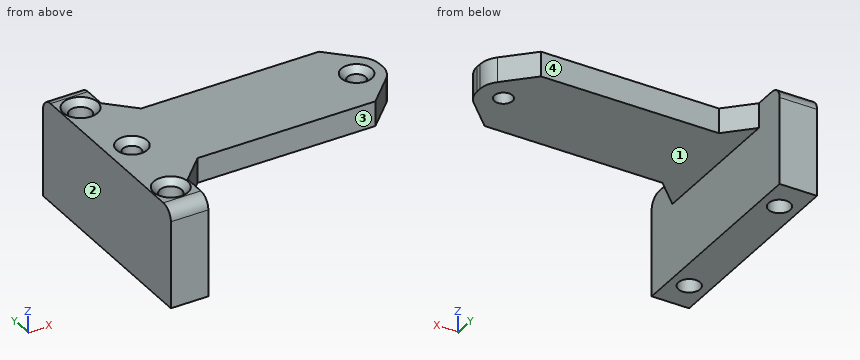
from build123d import *

# Parameters (mm, degrees)
SKETCH_W        = 6
SKETCH_H        = 34
PAD_DEPTH       = 12
PAD001_DEPTH    = 4
SKETCH003_R     = 1.75
POCKET_DEPTH    = 16.001
FILLET_R        = 2
CHAMFER_SIZE    = 1
SKETCH004_R     = 1.45
POCKET001_DEPTH = 6
CHAMFER001_SIZE = 5.5
FILLET001_R     = 4
CHAMFER002_SIZE = 4
CHAMFER003_SIZE = 1


with BuildPart() as part:
    # Sketch → Pad (new body)
    with BuildSketch(Plane.XY):
        with Locations((3, 17)):
            Rectangle(SKETCH_W, SKETCH_H)
    extrude(amount=PAD_DEPTH)

    # Sketch002 → Pad001 (join)
    with BuildSketch(Plane.XY.offset(12)):
        Polygon((6, 24.5), (44, 24.5), (44, 9.5), (6, 9.5), (6, 0), (0, 0), (0, 34), (6, 34), align=None)
    extrude(amount=PAD001_DEPTH)

    # Sketch003 (on Face11 of Pad001) → Pocket (cut, through all)
    with BuildSketch(Plane.XY.offset(16)):
        with Locations((3, 29)):
            Circle(SKETCH003_R)
        with Locations((3, 5)):
            Circle(SKETCH003_R)
    extrude(amount=-POCKET_DEPTH, mode=Mode.SUBTRACT)

    # Fillet
    fillet_edges = [part.edges().sort_by_distance(p)[0] for p in [
        (3, 0, 16),
        (3, 34, 16),
    ]]
    fillet(fillet_edges, radius=FILLET_R)

    # Chamfer
    chamfer_edges = [part.edges().sort_by_distance(p)[0] for p in [
        (1.25, 29, 16),
        (1.25, 5, 16),
    ]]
    chamfer(chamfer_edges, length=CHAMFER_SIZE)

    # Sketch004 (on Face1 of Chamfer) → Pocket001 (cut)
    with BuildSketch(Plane.XY.offset(16)):
        with Locations((4, 17)):
            Circle(SKETCH004_R)
        with Locations((40, 17)):
            Circle(SKETCH004_R)
    extrude(amount=-POCKET001_DEPTH, mode=Mode.SUBTRACT)

    # Chamfer001
    chamfer001_edges = [part.edges().sort_by_distance(p)[0] for p in [
        (44, 9.5, 14),
        (44, 24.5, 14),
    ]]
    chamfer(chamfer001_edges, length=CHAMFER001_SIZE)

    # Fillet001
    fillet001_edges = [part.edges().sort_by_distance(p)[0] for p in [
        (44, 15, 14),
        (44, 19, 14),
    ]]
    fillet(fillet001_edges, radius=FILLET001_R)

    # Chamfer002
    chamfer002_edges = [part.edges().sort_by_distance(p)[0] for p in [
        (6, 9.5, 14),
        (6, 24.5, 14),
    ]]
    chamfer(chamfer002_edges, length=CHAMFER002_SIZE)

    # Chamfer003
    chamfer003_edges = [part.edges().sort_by_distance(p)[0] for p in [
        (2.55, 17, 16),
        (38.55, 17, 16),
    ]]
    chamfer(chamfer003_edges, length=CHAMFER003_SIZE)


solid = part.part
The listing builds one solid part. Answer for the finished solid, in the listing's coordinates (mm). Face numbers are marked on the shaded views. A direction names the side the tool comes from. Round coordinates to 2 decimals unless told otherwise and drop trailing zeros. Order: outer loops, then holes, each group sorted by start corner. A loop starts at its lowest first (then second) coordinate and runs counter-clockwise, first axis right, second up. Notation, with made-up numbers: (-37, -23.75) -> (19, -23.75) arc R33 ccw to (19, 8.25) -> close; hole circle Ø8 at (83.25, 75.25). An arc over 180 degrees is marked (long way). Put each result on its own line as item: value.
Q1. Section C-C, the plane z = 10.5 is taken. Write down the section's boundary in (x, y), and give its area (3 significant figures).
Results list:
outline: (0, 0) -> (6, 0) -> (6, 34) -> (0, 34) -> close; hole circle Ø3.5 at (3, 5); hole circle Ø3.5 at (3, 29); hole circle Ø2.9 at (4, 17)
area: 178 mm^2
Q2. Consider line 1 along Y through (x, z) = (3, 12.75); line 2 along Y through (x, z) = (3, 6.25); line 3 along Y through (x, z) = (4, 11.75). Determine where each line is inside the solid, lowest interval first.
Results list:
line 1: 0 to 3.25, 6.75 to 15.95, 18.05 to 27.25, 30.75 to 34
line 2: 0 to 3.25, 6.75 to 27.25, 30.75 to 34
line 3: 0 to 3.56, 6.44 to 15.55, 18.45 to 27.56, 30.44 to 34
Q3. Section D-D, the plane z = 1.5 is taken. Write down the section's boundary in (x, y), and give its area (3 significant figures).
Results list:
outline: (0, 0) -> (6, 0) -> (6, 34) -> (0, 34) -> close; hole circle Ø3.5 at (3, 5); hole circle Ø3.5 at (3, 29)
area: 185 mm^2
Q4. Each of these flat-tipped pins is pushed along its axis until it touches: P1, Ø2, axis at x = 23, z = 15, coming from the -Y side; P2, Ø3.5, axis at x = 4, y = 17, coming from the +Z side; P3, Ø5.5, axis at x = 3, y = 29, coming from the -Z side; P4, Ø1.5, axis at y = 17, z = 6.5, coming from the +X side. Where does it stop, or does it pass through?
Results list:
P1: y = 9.5
P2: z = 15.3
P3: z = 0
P4: x = 6
Q5. Which of the six approach directions +Z, -Z, +X, -X, +Y, -Y give full straight-line access (tool end or side, diameter ignored) to the marked faces 1, 2, 3 and 4?
Results list:
face 1: -Z, +X, +Y, -Y
face 2: +Z, -Z, -X, +Y, -Y
face 3: +Z, -Z, +X, -Y
face 4: +Z, -Z, +X, +Y
Q6. Section B-B, the plane y = 29 is taken. Write down the section's boundary in (x, z), and give its area (3 significant figures).
Results list:
outline: (0, 0) -> (1.25, 0) -> (1.25, 15) -> (0.25, 16) -> (0, 16) -> close; (4.75, 0) -> (6, 0) -> (6, 16) -> (5.75, 16) -> (4.75, 15) -> close
area: 39.0 mm^2
Q7. Section A-A, the plane z = 13.25 is taken. Write down the section's boundary in (x, y).
Results list:
outline: (0, 0) -> (6, 0) -> (6, 5.5) -> (10, 9.5) -> (38.5, 9.5) -> (42.83, 13.83) arc R4 ccw to (44, 16.66) -> (44, 17.34) arc R4 ccw to (42.83, 20.17) -> (38.5, 24.5) -> (10, 24.5) -> (6, 28.5) -> (6, 34) -> (0, 34) -> close; hole circle Ø3.5 at (3, 5); hole circle Ø3.5 at (3, 29); hole circle Ø2.9 at (4, 17); hole circle Ø2.9 at (40, 17)
